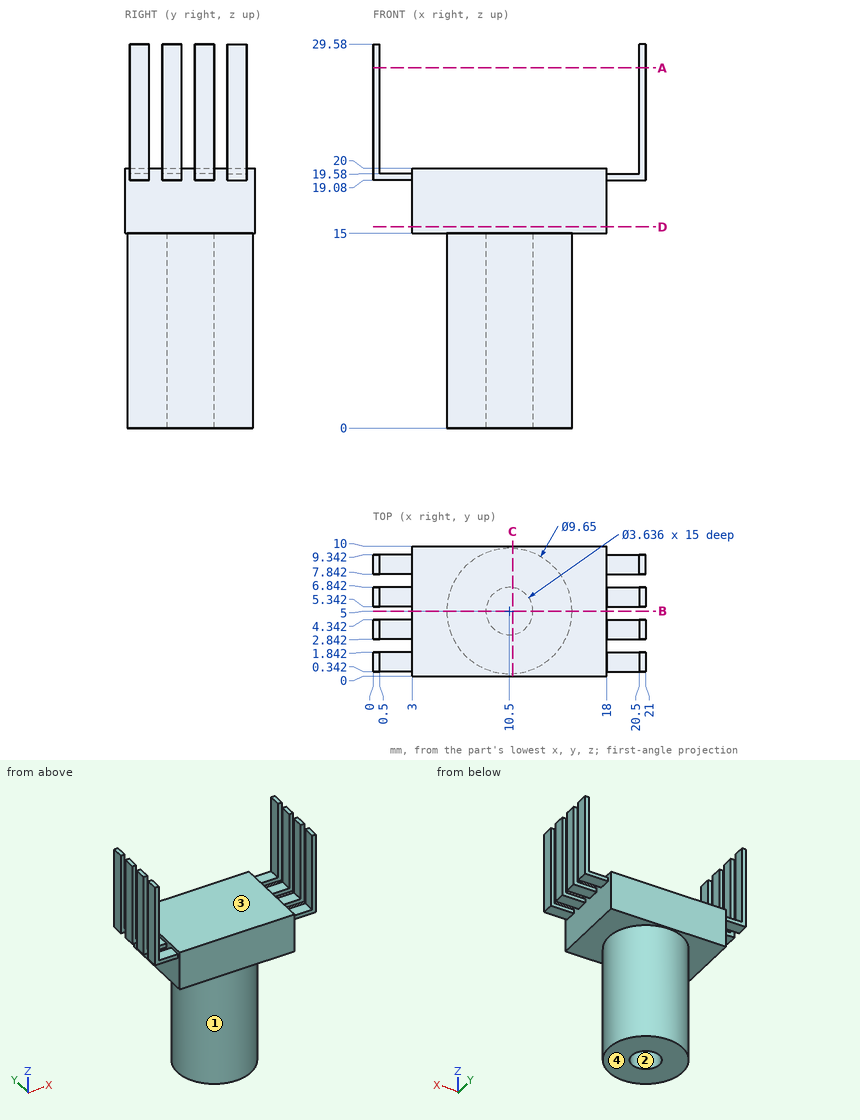
Here's the drawing with two shaded views (mm, measured from the low corner). I have some questions. Give positions to 0.01 mm unless a question says otherwise; leave off trailing zeros. Loops run counter-clockwise (first coordinate to the right, second up) from the corner with the lowest first, then second, coordinate; pieces in that order, holes last. Notation, with made-up numbers: (51.25, 70.25) - (62.25, 70.25) arc R17 cw to (62.25, 75.25) - close; hole circle Ø2 at (18, -39). An arc over 180 degrees is marked (long way). One line per item, written item: value.
(1) I need wall thicknesses on line 1 along Y through (x, z) = (10.5, 7.5) (1 decimal); line 2 along X through (y, z) = (6, 23.5); line 3 along Z through (x, y) = (8, 5.5). Which ranges of each line are inside material? Lowest first, please.
Verdict:
line 1: 0.2 to 3.2, 6.8 to 9.8
line 2: 0 to 0.5, 20.5 to 21
line 3: 0 to 20
(2) If we section it at A-A, the plane z = 27.75: State how many separate pieces and enclosed holes the cut face has.
Verdict:
separate pieces: 8
enclosed holes: 0
(3) If we section it at D-D, the plane z = 15.5: List the corners of the cut face in (x, y) for me, plus the area to 3 significant figures.
Verdict:
outline: (3, 0) - (18, 0) - (18, 10) - (3, 10) - close
area: 150 mm^2
(4) If we mould it in two halves opening along X, with no side actions, what happens to the marked faces 1, 2, 3 and 4? For each: released by +X, released by -X, zero draft, split by the parting line, or undercut.
Verdict:
face 1: split by the parting line
face 2: undercut
face 3: undercut
face 4: zero draft
(5) If we section it at B-B, the plane y = 5: List the corners of the cut face in (x, z) for me (1 decimal), plus the area to 3 significant figures.
Verdict:
outline: (3, 15) - (5.7, 15) - (5.7, 0) - (8.7, 0) - (8.7, 15) - (12.3, 15) - (12.3, 0) - (15.3, 0) - (15.3, 15) - (18, 15) - (18, 20) - (3, 20) - close
area: 165 mm^2
(6) If we section it at C-C, the plane x = 10.75: List the corners of the cut face in (y, z) for me.
Verdict:
outline: (0, 15) - (0.18, 15) - (0.18, 0) - (3.2, 0) - (3.2, 15) - (6.8, 15) - (6.8, 0) - (9.82, 0) - (9.82, 15) - (10, 15) - (10, 20) - (0, 20) - close
(7) I'm going to push flat-ended pins straight in: pin 1 (1.7 mm diameter, centred on x = 19.5, y = 0.5, fed in from -Z); pin 2 (2.5 mm diameter, centred on x = 1, z = 25.5, fed in from +Y); pin 3 (1 mm diameter, centred on y = 3.5, z = 3.5, fed in from +X). Where does each tip first touch, or does it pass through?
Verdict:
pin 1: z = 19.08
pin 2: y = 9.34
pin 3: x = 15.22
